Build history of the part. All positions in model axes, mm. Coordinates: 2 decimals unless noted, no trailing zeros. Loops run counter-clockwise (first coordinate to the right, second up) from the corner with the lowest first, then second, coordinate; pieces in that order, holes last.
Item 1: Flat gauge pins, fed straight in: pin 1 (0.5 mm diameter, centred on x = 0, z = -1, fed in from +Y); pin 2 (0.7 mm diameter, centred on y = 0, z = -0.5, fed in from +X); pin 3 (0.7 mm diameter, centred on y = 0, z = 0, fed in from -X); pin 4 (0.8 mm diameter, centred on x = 0.5, y = 0.5, fed in from +Z). Where does each tip first touch, or does it go through?
Item 2: Drill centre lines: line 1 along Z through (x, y) = (0.05, 1.15); line 2 along X through (y, z) = (0.05, -1). Where is each one in solid material? Low to high.
Item 3: Cut at B-B (z = -1). List the corners of the cut face in (x, y), and give its area (3 significant figures).
Item 4: Mould opens along X. For faces 1 (the face through (-1.25, 0, 2)), 2 (the face through (1.25, 0, 2)), 3 (the face through (0, 1, 3.5)) say: released by +X, released by -X, zero draft, split by the parting line, or undercut.
Item 5: Cut at A-A (x = -0.05). List the corners of the cut face in (y, z).
Item 6: Cut at C-C (y = -0.65). List the corners of the cut face in (x, z), and give its area (3 significant figures).
Autodesk Inventor part; units mm, degrees
ref_plane "YZ Plane" through (0, 0, 0) normal (1, 0, 0) x (0, 1, 0)
ref_plane "XZ Plane" through (0, 0, 0) normal (0, 1, 0) x (-1, 0, 0)
ref_plane "XY Plane" through (0, 0, 0) normal (0, 0, 1) x (1, 0, 0)
sketch "Sketch2" plane through (0, 0, 0) normal (0, 0, 1) x (1, 0, 0)
  line L0 (-0.3, 0.3) -> (0.3, 0.3)
  line L1 (0.3, 0.3) -> (0.3, -0.3)
  line L2 (0.3, -0.3) -> (-0.3, -0.3)
  line L3 (-0.3, -0.3) -> (-0.3, 0.3)
  line L4 (-0.3, 0.3) -> (0.3, -0.3) construction
  line L5 (0.3, 0.3) -> (-0.3, -0.3) construction
  point P0 (0, 0)
  dimension "d2" = 0.6
  dimension "d3" = 0.6
extrude "Extrusion1" add sketch "Sketch2" along normal blind 10 and the other way blind 2
sketch "Sketch3" plane through (0, 0, -2) normal (0, 0, -1) x (-1, 0, 0)
  line L0 (-0.3, -0.3) -> (0.3, -0.3)
  line L1 (0.3, -0.3) -> (0.3, 0.3)
  line L2 (0.3, 0.3) -> (-0.3, 0.3)
  line L3 (-0.3, 0.3) -> (-0.3, -0.3)
  line L4 (-1.25, 1.27) -> (1.25, 1.27)
  line L5 (1.25, 1.27) -> (1.25, -1.27)
  line L6 (1.25, -1.27) -> (-1.25, -1.27)
  line L7 (-1.25, -1.27) -> (-1.25, 1.27)
  line L8 (-1.25, 1.27) -> (1.25, -1.27) construction
  line L9 (1.25, 1.27) -> (-1.25, -1.27) construction
  point P0 (0, 0)
  dimension "d8" = 2.54
  dimension "d9" = 2.5
ref_plane "Work Plane1" through (0, 0, 1) normal (0, 0, -1) x (-1, 0, 0)
extrude "Extrusion2" add sketch "Sketch3" against normal blind 2.5 from surface at -3
properties part number "Header D1"
Filled sheet:
1. pin 1: stops at y = 0.3
1. pin 2: stops at x = 0.3
1. pin 3: stops at x = -0.3
1. pin 4: stops at z = 10
2. line 1: z = 1 to 3.5
2. line 2: x = -0.3 to 0.3
3. outline: (-0.3, -0.3) - (0.3, -0.3) - (0.3, 0.3) - (-0.3, 0.3) - close
3. area: 0.360 mm2
4. face 1: released by -X
4. face 2: released by +X
4. face 3: zero draft
5. outline: (-1.27, 1) - (-0.3, 1) - (-0.3, -2) - (0.3, -2) - (0.3, 1) - (1.27, 1) - (1.27, 3.5) - (0.3, 3.5) - (0.3, 10) - (-0.3, 10) - (-0.3, 3.5) - (-1.27, 3.5) - close
6. outline: (-1.25, 1) - (1.25, 1) - (1.25, 3.5) - (-1.25, 3.5) - close
6. area: 6.25 mm2
